```python
from build123d import *

# Parameters (mm, degrees)
SKETCH1_R           = 6.35
BOSS_EXTRUDE1_DEPTH = 3.175
SKETCH2_R           = 6.35
SKETCH2_R_2         = 3.175
BOSS_EXTRUDE2_DEPTH = 6.35
CUT_EXTRUDE2_DEPTH  = 6.35
SKETCH5_W           = 6.35
SKETCH5_H           = 12.7
BOSS_EXTRUDE3_DEPTH = 12.7
SKETCH6_W           = 6.35
SKETCH6_H           = 12.7
BOSS_EXTRUDE4_DEPTH = 5.08
SKETCH7_R           = 6.35
BOSS_EXTRUDE5_DEPTH = 6.35
SKETCH9_W           = 12.7
SKETCH9_H           = 12.7
CUT_EXTRUDE4_DEPTH  = 3.175


with BuildPart() as part:
    # Sketch1 → Boss-Extrude1 (new body, symmetric)
    with BuildSketch(Plane.XY):
        with BuildLine():
            Line((7.099515829, 6.35), (31.75, 6.35))
            Line((31.75, 6.35), (36.83, 6.35))
            Line((36.83, 6.35), (36.83, -6.35))
            Line((36.83, -6.35), (31.75, -6.35))
            Line((31.75, -6.35), (7.099515829, -6.35))
            ThreePointArc((7.099515829, -6.35), (0, -9.525), (-7.099515829, -6.35))
            Line((-7.099515829, -6.35), (-17.78, -6.35))
            Line((-17.78, -6.35), (-17.78, 6.35))
            Line((-17.78, 6.35), (-7.099515829, 6.35))
            ThreePointArc((-7.099515829, 6.35), (0, 9.525), (7.099515829, 6.35))
        make_face()
        Circle(SKETCH1_R, mode=Mode.SUBTRACT)
    extrude(amount=BOSS_EXTRUDE1_DEPTH, both=True)

    # Sketch2 → Boss-Extrude2 (add)
    with BuildSketch(Plane(origin=(0, 0, -3.175), x_dir=(-1, 0, 0), z_dir=(0, 0, -1))):
        with Locations((-36.83, 0)):
            Circle(SKETCH2_R)
        with Locations((-36.83, 0)):
            Circle(SKETCH2_R_2, mode=Mode.SUBTRACT)
    extrude(amount=-BOSS_EXTRUDE2_DEPTH)

    # Sketch4 → Cut-Extrude2 (cut)
    with BuildSketch(Plane.XY.offset(3.175)):
        with BuildLine():
            Line((36.83, 3.175), (17.78, 3.175))
            ThreePointArc((17.78, 3.175), (14.605, 0), (17.78, -3.175))
            Line((17.78, -3.175), (36.83, -3.175))
            ThreePointArc((36.83, -3.175), (40.005, 0), (36.83, 3.175))
        make_face()
    extrude(amount=-CUT_EXTRUDE2_DEPTH, mode=Mode.SUBTRACT)

    # Sketch5 → Boss-Extrude3 (add)
    with BuildSketch(Plane.XY.offset(3.175)):
        with Locations((-14.605, 0)):
            Rectangle(SKETCH5_W, SKETCH5_H)
    extrude(amount=BOSS_EXTRUDE3_DEPTH)

    # Sketch6 → Boss-Extrude4 (add)
    with BuildSketch(Plane.ZY.offset(17.78)):
        with Locations((12.7, 0)):
            Rectangle(SKETCH6_W, SKETCH6_H)
    extrude(amount=BOSS_EXTRUDE4_DEPTH)

    # Sketch7 → Boss-Extrude5 (add)
    with BuildSketch(Plane.XY.offset(15.875)):
        with Locations((-22.86, 0)):
            Circle(SKETCH7_R)
    extrude(amount=-BOSS_EXTRUDE5_DEPTH)

    # Sketch9 → Cut-Extrude4 (cut)
    with BuildSketch(Plane.ZY.offset(17.78)):
        with Locations((3.175, 0)):
            Rectangle(SKETCH9_W, SKETCH9_H)
    extrude(amount=-CUT_EXTRUDE4_DEPTH, mode=Mode.SUBTRACT)


solid = part.part
```
Verification items for the finished model (mm, model axes). A direction names the side the tool comes from. Give positions to 0.01 mm unless a question says otherwise; leave off trailing zeros. Order: outer loops, then holes, each group sorted by start corner. A loop starts at its lowest first (then second) coordinate and runs counter-clockwise, first axis right, second up. Notation, with made-up numbers: M 60.5,88.25 L 92.5,88.25 A3 ccw 92.5,92.25 Z; hole C 11.25,59 d7. An arc over 180 degrees is marked long. Answer in a Markdown table with one row per item. Add a question column.
Item 1: Scan lines: probe 1 along Y at (x, z) = (0, 1.5) (3 decimals); probe 2 along Z at (x, y) = (-10, 0) (3 decimals); probe 3 along X at (y, z) = (-2, 7) (3 decimals). Record each from-to range of solid material in increasing order. Write a range as from..to.
Item 2: Section check C-C, the plane y = -1. Enter the section's corners in (x, z) (3 decimals), and give its area (3 significant figures).
Item 3: Mould release check, pull along X, two halves, no side actions. Record for faces 1 (the flat face through (22, -6.35, 0)), 2 (the flat face through (-11.43, 0, 9)), 3 (the cylindrical face through (40.004, 0.07, -0.044)): released by +X, released by -X, zero draft, split by the parting line, or undercut.
Item 4: Tool access check on faces 4 (the cylindrical face through (14.606, 0.07, 0.044)), 5 (the flat face through (-14.605, 0, 3)), 6 (the flat face through (-13, -6.35, 8)), 7 (the flat face through (-13, 6.35, 8)). Record the directions out of +Z, -Z, +X, -X, +Y, -Y that give a thin tool (end or side, any length) a straight path to the whole face; none if there is none.
Item 5: Section check D-D, the plane y = -4. Enter the section's corners in (x, z) (3 decimals).
Item 6: Section check A-A, the plane x = 1. Enter the section's corners in (y, z) (3 decimals).
Item 7: Section check B-B, the plane z = 1.25. Enter the section's corners in (x, y) (3 decimals).
Item 8: Gauge pin test, flat ends, axial feed: pin 1 (6 mm diameter, centred on y = -4.5, z = 12, fed in from -X); pin 2 (6 mm diameter, centred on y = -6.5, z = 3.5, fed in from +X); pin 3 (10 mm diameter, centred on x = -9, z = 9.5, fed in from -Y). Record the tip position at first contact, or that the pin passes through.
Filled sheet:
| question | item | result |
|---|---|---|
| 1 | probe 1 | y = -9.525..-6.35, 6.35..9.525 |
| 1 | probe 2 | z = -3.175..3.175 |
| 1 | probe 3 | x = -14.605..-11.43 |
| 2 | outline | M -29.131,9.525 L -14.605,9.525 L -14.605,-3.175 L -6.271,-3.175 L -6.271,3.175 L -11.43,3.175 L -11.43,15.875 L -29.131,15.875 Z; M 6.271,-3.175 L 14.767,-3.175 L 14.767,3.175 L 6.271,3.175 Z; M 39.843,-3.175 L 43.101,-3.175 L 43.101,3.175 L 39.843,3.175 Z |
| 2 | area | 260 mm^2 |
| 3 | face 1 | zero draft |
| 3 | face 2 | released by +X |
| 3 | face 3 | undercut |
| 4 | face 4 | +Z, -Z |
| 4 | face 5 | -Z, -X, +Y, -Y |
| 4 | face 6 | +Z, -Z, -X, -Y |
| 4 | face 7 | +Z, -Z, -X, +Y |
| 5 | outline | M -27.792,9.525 L -14.605,9.525 L -14.605,-3.175 L -4.932,-3.175 L -4.932,3.175 L -11.43,3.175 L -11.43,15.875 L -27.792,15.875 Z; M 4.932,-3.175 L 41.762,-3.175 L 41.762,3.175 L 4.932,3.175 Z |
| 6 | outline | M -9.472,-3.175 L -6.271,-3.175 L -6.271,3.175 L -9.472,3.175 Z; M 6.271,-3.175 L 9.472,-3.175 L 9.472,3.175 L 6.271,3.175 Z |
| 7 | outline | M -14.605,-6.35 L -7.1,-6.35 A9.525 ccw 7.1,-6.35 L 36.83,-6.35 A6.35 ccw 36.83,6.35 L 7.1,6.35 A9.525 ccw -7.1,6.35 L -14.605,6.35 Z; hole C 0,0 d12.7; hole M 17.78,-3.175 L 36.83,-3.175 A3.175 ccw 36.83,3.175 L 17.78,3.175 A3.175 ccw Z |
| 8 | pin 1 | stops at x = -29.03 |
| 8 | pin 2 | stops at x = 42.12 |
| 8 | pin 3 | stops at y = -6.35 |
